Could you check a few things on this model? Use its own coordinates, in mm. A direction names the side the tool comes from. Coordinates: 2 decimals unless noted, no trailing zeros. Loops run counter-clockwise (first coordinate to the right, second up) from the corner with the lowest first, then second, coordinate; pieces in that order, holes last. Notation, with made-up numbers: (30, 5) -> (82, 5) arc R22 ccw to (82, 25) -> close; hole circle Ø10 at (-2, -23.5). An arc over 180 degrees is marked (long way). One line per question, with ' | ' between items.
```python
from build123d import *

# Parameters (mm, degrees)
SKETCH1_W               = 88
SKETCH1_H               = 110
SKETCH1_R               = 5
BOSS_EXTRUDE1_DEPTH     = 24
SKETCH3_R               = 9.5
BOSS_EXTRUDE2_DEPTH     = 12
FILLET1_R               = 5
SKETCH4_W               = 88
SKETCH4_H               = 6
CUT_EXTRUDE1_DEPTH      = 35
FILLET2_R               = 3
SKETCH5_R               = 23
CUT_EXTRUDE2_DEPTH      = 109
CUT_EXTRUDE2_DEPTH_BACK = 35


with BuildPart() as part:
    # Sketch1 → Boss-Extrude1 (new body)
    with BuildSketch(Plane(origin=(0, 0, 0), x_dir=(1, 0, 0), z_dir=(0, 1, 0))):
        with Locations((0, 55)):
            Rectangle(SKETCH1_W, SKETCH1_H)
        with Locations((-27.5, 95)):
            Circle(SKETCH1_R, mode=Mode.SUBTRACT)
        with Locations((-27.5, 60)):
            Circle(SKETCH1_R, mode=Mode.SUBTRACT)
        with Locations((27.5, 60)):
            Circle(SKETCH1_R, mode=Mode.SUBTRACT)
        with Locations((27.5, 95)):
            Circle(SKETCH1_R, mode=Mode.SUBTRACT)
    extrude(amount=-BOSS_EXTRUDE1_DEPTH)

    # Sketch3 → Boss-Extrude2 (add)
    with BuildSketch(Plane.XY):
        with BuildLine():
            Line((-44, -24), (-19.769224603, -55.302867659))
            ThreePointArc((-19.769224603, -55.302867659), (0, -65), (19.769224603, -55.302867659))
            Line((19.769224603, -55.302867659), (44, -24))
            Line((44, -24), (-44, -24))
        make_face()
        with Locations((0, -40)):
            Circle(SKETCH3_R, mode=Mode.SUBTRACT)
    extrude(amount=-BOSS_EXTRUDE2_DEPTH)

    # Fillet1
    fillet1_edges = [part.edges().sort_by_distance(p)[0] for p in [
        (-44, 0, -55),
        (44, 0, -55),
    ]]
    fillet(fillet1_edges, radius=FILLET1_R)

    # Sketch4 → Cut-Extrude1 (cut)
    with BuildSketch(Plane(origin=(0, 0, -110), x_dir=(-1, 0, 0), z_dir=(0, 0, -1))):
        with Locations((0, -21)):
            Rectangle(SKETCH4_W, SKETCH4_H)
    extrude(amount=-CUT_EXTRUDE1_DEPTH, mode=Mode.SUBTRACT)

    # Fillet2
    fillet2_edges = [part.edges().sort_by_distance(p)[0] for p in [
        (0, -18, -75),
    ]]
    fillet(fillet2_edges, radius=FILLET2_R)

    # Sketch5 → Cut-Extrude2 (cut, two sides)
    with BuildSketch(Plane(origin=(0, 0, 0), x_dir=(1, 0, 0), z_dir=(0, 0.422618262, -0.906307787))) as cut_extrude2_sk:
        Circle(SKETCH5_R)
    extrude(amount=CUT_EXTRUDE2_DEPTH, mode=Mode.SUBTRACT)
    extrude(cut_extrude2_sk.sketch, amount=-CUT_EXTRUDE2_DEPTH_BACK, mode=Mode.SUBTRACT)


solid = part.part
```
Q1. Please list where these lines run through material, in increasing order: L1, parallel to X at y = -12.5, z = -60; L2, parallel to Z at x = -27.5, y = -11; L3, parallel to X at y = -11.5, z = -57.5. Write a range as [from, to].
Values follow:
L1: x = [-44, -32.5], [-22.5, 22.5], [32.5, 44] | L2: z = [-110, -100], [-90, -65], [-55, 0] | L3: x = [-44, -31.83], [-23.17, 23.17], [31.83, 44]
Q2. Imagine slicing it at C-C on y = -40. Write out the boundary of the cut face in (x, z).
Values follow:
outline: (-31.61, -12) -> (-9.5, -12) -> (-9.5, 0) -> (-31.61, 0) -> close; (9.5, -12) -> (31.61, -12) -> (31.61, 0) -> (9.5, 0) -> close
Q3. Imagine slicing it at B-B on x = 26. Write out the boundary of the cut face in (y, z), plus the area to 3 significant figures.
Values follow:
outline: (-47.25, -12) -> (-24, -12) -> (-24, -55.23) -> (0, -55.23) -> (0, 0) -> (-47.25, 0) -> close; (-24, -75) -> (-21, -75) arc R3 cw to (-18, -78) -> (-18, -90.23) -> (0, -90.23) -> (0, -64.77) -> (-24, -64.77) -> close; (-18, -110) -> (0, -110) -> (0, -99.77) -> (-18, -99.77) -> close | area: 2,310 mm2
Q4. For pin 1 (1 mm diameter, centred on x = -30, y = -33.5, fed in from -Z); pin 2 (8 mm diameter, centred on x = -27.5, z = -60, fed in from +Y); pin 3 (6 mm diameter, centred on x = -10.5, z = -31, fed in from +Y); pin 4 (1.5 mm diameter, centred on x = 21.5, y = -23, fed in from -Z), each with a flat end and sliding along its axis, tell me the tip position at first contact or that it passes through.
Values follow:
pin 1: stops at z = -12 | pin 2: passes through | pin 3: stops at y = -5.7 | pin 4: stops at z = -75
Q5. Imagine slicing it at A-A on z = -60. Write out the boundary of the cut face in (x, y), plus the area to 3 significant figures.
Values follow:
outline: (-44, -24) -> (-32.5, -24) -> (-32.5, 0) -> (-39, 0) arc R5 ccw to (-44, -5) -> close; (-22.5, -24) -> (22.5, -24) -> (22.5, 0) -> (-22.5, 0) -> close; (32.5, -24) -> (44, -24) -> (44, -5) arc R5 ccw to (39, 0) -> (32.5, 0) -> close | area: 1,620 mm2
Q6. We'd pull the mould along Z, two halves only. Please class faces 1 (the face through (-31.185, -11.832, -63.379)), 2 (the face through (23.815, -11.832, -63.379)), 3 (the face through (1, -18, -94)), 4 (the face through (-10, -32, 0)): released by +Z, released by -Z, zero draft, split by the parting line, or undercut.
Values follow:
face 1: undercut | face 2: undercut | face 3: zero draft | face 4: released by +Z
Q7. Imagine slicing it at D-D on z = -95. Write out the boundary of the cut face in (x, y).
Values follow:
outline: (-44, -18) -> (-32.5, -18) -> (-32.5, 0) -> (-39, 0) arc R5 ccw to (-44, -5) -> close; (-22.5, -18) -> (22.5, -18) -> (22.5, 0) -> (-22.5, 0) -> close; (32.5, -18) -> (44, -18) -> (44, -5) arc R5 ccw to (39, 0) -> (32.5, 0) -> close
Q8. For faces 5 (the face through (31.715, -39.871, -5.916)), 6 (the face through (9, -44, -12)), which set-ups out of +Z, -Z, +X, -X, +Y, -Y let a thin tool reach every point of the face, with its end or its side?
Values follow:
face 5: +Z, -Z, +X, -Y | face 6: -Z, +X, -X, -Y
